```python
from build123d import *

# Parameters (mm, degrees)
SKETCH1_W           = 2
SKETCH1_H           = 3
SKETCH1_R           = 2
SKETCH1_R_2         = 1.25
BOSS_EXTRUDE1_DEPTH = 15
SKETCH1_3_W         = 2
SKETCH1_3_H         = 3
SKETCH1_3_R         = 2
SKETCH1_3_R_2       = 1.25
BOSS_EXTRUDE2_DEPTH = 1
BOSS_EXTRUDE3_START = 15
SKETCH1_4_R         = 1.25
BOSS_EXTRUDE3_DEPTH = 3


with BuildPart() as part:
    # Sketch1 → Boss-Extrude1 (new body)
    # profile 1 of 5: a face of its own
    with BuildSketch(Plane(origin=(0, 0, 0), x_dir=(1, 0, 0), z_dir=(0, 1, 0))):
        with BuildLine():
            Line((3, 4), (-3, 4))
            ThreePointArc((-3, 4), (-5, 0), (-3, -4))
            Line((-3, -4), (3, -4))
            ThreePointArc((3, -4), (4.472135955, -2.236067977), (5, 0))
            ThreePointArc((5, 0), (4.472135955, 2.236067977), (3, 4))
        make_face()
        with Locations((-3.4375, 0)):
            Rectangle(SKETCH1_W, SKETCH1_H, mode=Mode.SUBTRACT)
        Circle(SKETCH1_R, mode=Mode.SUBTRACT)
        with Locations((3.4375, 0)):
            Rectangle(SKETCH1_W, SKETCH1_H, mode=Mode.SUBTRACT)
    # profile 2 of 5: a face of its own
    with BuildSketch(Plane(origin=(0, 0, 0), x_dir=(1, 0, 0), z_dir=(0, 1, 0))):
        with Locations((-3.4375, 0)):
            Rectangle(SKETCH1_W, SKETCH1_H)
    # profile 3 of 5: a face of its own
    with BuildSketch(Plane(origin=(0, 0, 0), x_dir=(1, 0, 0), z_dir=(0, 1, 0))):
        Circle(SKETCH1_R)
        Circle(SKETCH1_R_2, mode=Mode.SUBTRACT)
    # profile 4 of 5: a face of its own
    with BuildSketch(Plane(origin=(0, 0, 0), x_dir=(1, 0, 0), z_dir=(0, 1, 0))):
        Circle(SKETCH1_R_2)
    # profile 5 of 5: a face of its own
    with BuildSketch(Plane(origin=(0, 0, 0), x_dir=(1, 0, 0), z_dir=(0, 1, 0))):
        with Locations((3.4375, 0)):
            Rectangle(SKETCH1_W, SKETCH1_H)
    extrude(amount=BOSS_EXTRUDE1_DEPTH)

    # Sketch1<3> → Boss-Extrude2 (add)
    # profile 1 of 4: a face of its own
    with BuildSketch(Plane(origin=(0, 0, 0), x_dir=(1, 0, 0), z_dir=(0, 1, 0))):
        with Locations((-3.4375, 0)):
            Rectangle(SKETCH1_3_W, SKETCH1_3_H)
    # profile 2 of 4: a face of its own
    with BuildSketch(Plane(origin=(0, 0, 0), x_dir=(1, 0, 0), z_dir=(0, 1, 0))):
        with Locations((3.4375, 0)):
            Rectangle(SKETCH1_3_W, SKETCH1_3_H)
    # profile 3 of 4: a face of its own
    with BuildSketch(Plane(origin=(0, 0, 0), x_dir=(1, 0, 0), z_dir=(0, 1, 0))):
        with Locations(Location((0, 0, 0), (0, 0, 270))):
            Circle(SKETCH1_3_R)
        Circle(SKETCH1_3_R_2, mode=Mode.SUBTRACT)
    # profile 4 of 4: a face of its own
    with BuildSketch(Plane(origin=(0, 0, 0), x_dir=(1, 0, 0), z_dir=(0, 1, 0))):
        Circle(SKETCH1_3_R_2)
    extrude(amount=-BOSS_EXTRUDE2_DEPTH)

    # Sketch1<4> → Boss-Extrude3 (add)
    with BuildSketch(Plane(origin=(0, 0, 0), x_dir=(1, 0, 0), z_dir=(0, 1, 0)).offset(BOSS_EXTRUDE3_START)):
        with Locations(Location((0, 0, 0), (0, 0, 270))):
            Circle(SKETCH1_4_R)
    extrude(amount=BOSS_EXTRUDE3_DEPTH)


solid = part.part
```
Build history of the part. All positions in model axes, mm. A direction names the side the tool comes from. Coordinates: 2 decimals unless noted, no trailing zeros. Order: outer loops, then holes, each group sorted by start corner. A loop starts at its lowest first (then second) coordinate and runs counter-clockwise, first axis right, second up. Notation, with made-up numbers: M 78.25,22.25 L 135.25,22.25 A26 ccw 135.25,36.25 Z; hole C 5,86.5 d11. An arc over 180 degrees is marked long. One line per question, with ' | ' between items. Start each with the question number.
1. Wall check: line 1 along Z through (x, y) = (4, 13.25); line 2 along Y through (x, z) = (-1.75, -1.5); line 3 along Y through (x, z) = (-3, 0). Give the ranges that are in metal, low to high. Write a range as [from, to].
2. Tool access for faces 4 (the face through (4.438, -0.5, 0)), 5 (the face through (-4.438, -0.5, 0)), 6 (the face through (-2.438, -0.5, 0)), 7 (the face through (-3.5, -0.5, 1.5)), 8 (the face through (1, 15, -1)): list every direction of +Z, -Z, +X, -X, +Y, -Y with a clear straight run to the whole face (end or side of a thin tool).
3. Cut at C-C (y = 16.5). Write the cut outline in (x, z), plus the area to 3 significant figures.
4. Cut at A-A (y = 11). Write the cut outline in (x, z).
5. Cut at B-B (x = -1.5). Write the cut outline in (y, z), plus the area to 3 significant figures.
6. Mould opens along X. For faces 1 (the face through (0, -1, 0)), 2 (the face through (2.438, -0.5, 0)), 3 (the face through (-5, 7, 0)) say: +X half, -X half, draft (parallel to the pull), parting line (faces both ways), or undercut.
7. Flat gauge pins, fed straight in: P1, Ø0.5, axis at x = -3.5, y = -0.5, coming from the -Z side; P2, Ø0.8, axis at y = -0.5, z = 0, coming from the +X side; P3, Ø0.5, axis at x = 3, y = -0.5, coming from the +Z side. Where does each tip first touch, or does it go through?
The answers:
1) line 1: z = [-3, 3] | line 2: y = [0, 15] | line 3: y = [-1, 15]
2) face 4: +Z, -Z, +X, -Y | face 5: +Z, -Z, -X, -Y | face 6: +Z, -Z, -Y | face 7: +Z, -X, -Y | face 8: +Y
3) outline: C 0,0 d2.5 | area: 4.91 mm2
4) outline: M -3,-4 L 3,-4 A5 ccw 3,4 L -3,4 A5 ccw Z
5) outline: M -1,-1.32 L 0,-1.32 L 0,-4 L 15,-4 L 15,4 L 0,4 L 0,1.32 L -1,1.32 Z | area: 123 mm2
6) face 1: draft | face 2: undercut | face 3: -X half
7) P1: stops at z = -1.5 | P2: stops at x = 4.44 | P3: stops at z = 1.5
